Geometry check sheet. Reference: the model listing, model coordinates, mm. Round coordinates to 2 decimals unless told otherwise and drop trailing zeros. Write each loop counter-clockwise with the first axis right and the second up, starting at its lowest first coordinate (ties: lowest second). Pieces come first, ordered by that corner, then holes. Notation, with made-up numbers: (-8, 23.25) -> (32, 23.25) arc R16 cw to (32, 44.25) -> close; hole circle Ø9 at (20, 78.5). An arc over 180 degrees is marked (long way). One line per question, with ' | ' between items.
```python
from build123d import *

# Parameters (mm, degrees)
SKETCH1_R               = 7.6
SKETCH1_R_2             = 5
SKETCH1_W               = 10
SKETCH1_H               = 3.15
BOSS_EXTRUDE1_DEPTH     = 3
FILLET1_R               = 10
SKETCH2_W               = 3.2
SKETCH2_H               = 6
SKETCH2_H_2             = 2.5
SKETCH2_W_2             = 1
SKETCH2_H_3             = 2
CUT_EXTRUDE1_DEPTH      = 1
CUT_EXTRUDE1_DEPTH_BACK = 4


with BuildPart() as part:
    # Sketch1 → Boss-Extrude1 (new body)
    with BuildSketch(Plane(origin=(0, 0, 0), x_dir=(0, 0, -1), z_dir=(1, 0, 0))):
        Polygon((102.223805307, 6), (123.223805307, 6), (102.223805307, 27), align=None)
        Polygon((102.223805307, 6), (123.223805307, 6), (123.223805307, -9), (107.223805307, -9), (107.223805307, 0), (30, 0), (30, -9), (12.5, -9), (12.5, 0), (0, 0), (0, 46), (20.444761061, 46), (20.444761061, 43), (40.889522123, 43), (40.889522123, 46), (61.334283184, 46), (61.334283184, 43), (81.779044246, 43), (81.779044246, 46), (102.223805307, 46), align=None)
        with Locations((84.723805307, 21)):
            Circle(SKETCH1_R, mode=Mode.SUBTRACT)
        with Locations((51.111902654, 17.95)):
            Circle(SKETCH1_R, mode=Mode.SUBTRACT)
        with Locations((17.5, 14.9)):
            Circle(SKETCH1_R_2, mode=Mode.SUBTRACT)
        with Locations((115.223805307, -4.575)):
            Rectangle(SKETCH1_W, SKETCH1_H, mode=Mode.SUBTRACT)
        with Locations((21.25, -4.575)):
            Rectangle(SKETCH1_W, SKETCH1_H, mode=Mode.SUBTRACT)
    extrude(amount=BOSS_EXTRUDE1_DEPTH)

    # Fillet1
    fillet1_edges = [part.edges().sort_by_distance(p)[0] for p in [
        (1.5, 6, -123.223805307),
        (1.5, 27, -102.223805307),
    ]]
    fillet(fillet1_edges, radius=FILLET1_R)

    # Sketch2 → Cut-Extrude1 (cut, two sides)
    with BuildSketch(Plane(origin=(3, 0, 0), x_dir=(0, 0, -1), z_dir=(1, 0, 0))) as cut_extrude1_sk:
        with Locations((51.111902654, 38.5)):
            Rectangle(SKETCH2_W, SKETCH2_H)
        with Locations((51.111902654, 42.75)):
            Rectangle(SKETCH2_W, SKETCH2_H_2)
        with Locations((49.011902654, 42.75)):
            Rectangle(SKETCH2_W_2, SKETCH2_H_2)
        with Locations((51.111902654, 45)):
            Rectangle(SKETCH2_W, SKETCH2_H_3)
        with Locations((53.211902654, 42.75)):
            Rectangle(SKETCH2_W_2, SKETCH2_H_2)
    extrude(amount=CUT_EXTRUDE1_DEPTH, mode=Mode.SUBTRACT)
    extrude(cut_extrude1_sk.sketch, amount=-CUT_EXTRUDE1_DEPTH_BACK, mode=Mode.SUBTRACT)


solid = part.part
```
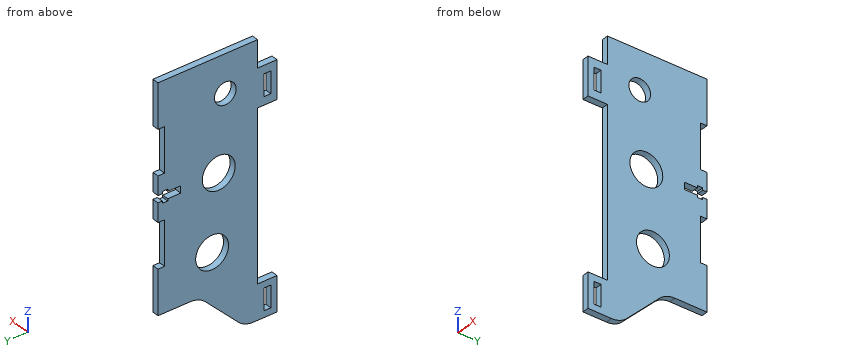
(1) Material ranges on line 1 (Y direction, x = 2.1, z = -17.5); line 2 (Z direction, x = 2.65, y = 15.5); line 3 (Y direction, x = 0.55, z = -100), recorded low to high.
Resolved:
line 1: y = -9 to -6.15, -3 to 9.9, 19.9 to 46 | line 2: z = -113.72 to -89.97, -79.48 to -58.31, -43.92 to -22.46, -12.54 to 0 | line 3: y = 0 to 46
(2) Sectioned sample at B-B on y = -1.5. Record the cut outline in (x, z), then the cut area to 4 significant figures.
Resolved:
outline: (0, -123.22) -> (3, -123.22) -> (3, -107.22) -> (0, -107.22) -> close; (0, -30) -> (3, -30) -> (3, -12.5) -> (0, -12.5) -> close | area: 100.5 mm2
(3) Go/stop test with flat-tipped pins: pin 1 (0.9 mm diameter, centred on x = 1, z = -6, fed in from -Y); pin 2 (0.9 mm diameter, centred on x = 2, z = -51, fed in from +Y); pin 3 (1.5 mm diameter, centred on x = 2, y = -6.5, fed in from +Z). Record where each tip stops, or that it passes through.
Resolved:
pin 1: stops at y = 0 | pin 2: stops at y = 35.5 | pin 3: stops at z = -12.5
(4) Sectioned sample at C-C on y = 21. Record the cut outline in (x, z), then the cut area to 3 significant figures.
Resolved:
outline: (0, -108.22) -> (3, -108.22) -> (3, -92.32) -> (0, -92.32) -> close; (0, -77.12) -> (3, -77.12) -> (3, -58.07) -> (0, -58.07) -> close; (0, -44.15) -> (3, -44.15) -> (3, 0) -> (0, 0) -> close | area: 237 mm2
(5) Sectioned sample at A-A on z = -17.5. Record the cut outline in (x, y).
Resolved:
outline: (0, -9) -> (3, -9) -> (3, -6.15) -> (0, -6.15) -> close; (0, -3) -> (3, -3) -> (3, 9.9) -> (0, 9.9) -> close; (0, 19.9) -> (3, 19.9) -> (3, 46) -> (0, 46) -> close
(6) Sectioned sample at D-D on z = -111.5. Record the cut outline in (x, y), then the cut area to 3 significant figures.
Resolved:
outline: (0, -9) -> (3, -9) -> (3, -6.15) -> (0, -6.15) -> close; (0, -3) -> (3, -3) -> (3, 17.72) -> (0, 17.72) -> close | area: 70.7 mm2
